Here's how the part is built. I have some questions about the finished solid (model axes, mm). Face numbers are marked on the shaded views. A direction names the side the tool comes from. Coordinates: 2 decimals unless noted, no trailing zeros. Loops run counter-clockwise (first coordinate to the right, second up) from the corner with the lowest first, then second, coordinate; pieces in that order, holes last. Notation, with made-up numbers: (0.5, -18) -> (41.5, -18) arc R9 cw to (41.5, -3) -> close; hole circle Ø7 at (42, 24). An arc over 180 degrees is marked (long way). Answer as a JSON object with one key per item and string values. Group by question number.
1) I need wall thicknesses on probe 1 along X at (y, z) = (-31, 39); probe 2 along Y at (x, z) = (14, 156.5); probe 3 along Y at (x, z) = (12, 41.5). Which ranges of each line are inside material? Lowest first, please. Write a range as [from, to].
2) I want a section at A-A (z = 48). Write out the boundary of the cut face in (x, y).
3) If we mould it in two halves opening along Y, with no side actions, what happens to the marked faces 1, 2 and 3? For each: +Y half, -Y half, draft (parallel to the pull), parting line (faces both ways), or undercut.
4) Which directions (+Z, -Z, +X, -X, +Y, -Y) give clear straight access to the entire face, cutting with the end or side of a thin tool? Please do the marked faces 4 and 5.
5) I want a section at B-B (x = 20). Write out the boundary of the cut face in (y, z), then the cut area to 3 significant figures.
6) I want a section at D-D (x = 38). Write out the boundary of the cut face in (y, z), then the cut area to 3 significant figures.
7) I want a section at C-C (y = 32). Write out the boundary of the cut face in (x, z), then the cut area to 4 significant figures.
8) I'm going to push a flat-ended pin straight in: pin 1 (10 mm diameter, centred on y = 1, z = 142, fed in from +X). Where does the tip first touch, or does it pass through?
Autodesk Inventor part; units mm, degrees
ref_plane "Начальная плоскость" through (0, 0, 23) normal (0, 0, 1) x (1, 0, 0)
ref_plane "Конечная плоскость" through (0, 0, 232) normal (0, 0, 1) x (1, 0, 0)
ref_plane "РабПлоскость8" through (-82, -50, 23) normal (0, 0, -1) x (-1, 0, 0)
ref_plane "Начальная плоскость" through (0, 0, 23) normal (0, 0, 1) x (1, 0, 0)
ref_plane "Конечная плоскость" through (0, 0, 232) normal (0, 0, 1) x (1, 0, 0)
sketch "Эскиз" plane through (0, 0, 0) normal (0, 0, 1) x (1, 0, 0)
  line L0 (46, -50) -> (0, -50)
  line L1 (46, -50) -> (46, -46.6496)
  line L2 (43.2392, -43.6591) -> (10.9418, -41.0753)
  line L3 (4.5, -34.0976) -> (4.5, 34.0976)
  line L4 (43.2392, 43.6591) -> (10.9418, 41.0753)
  line L5 (46, 46.6496) -> (46, 50)
  line L6 (0, 50) -> (46, 50)
  line L7 (0, -50) -> (0, 50)
  arc A0 (4.5, -34.0976) -> (10.9418, -41.0753) centre (11.5, -34.0976) ccw
  arc A1 (10.9418, 41.0753) -> (4.5, 34.0976) centre (11.5, 34.0976) ccw
  arc A2 (46, -46.6496) -> (43.2392, -43.6591) centre (43, -46.6496) ccw
  arc A3 (43.2392, 43.6591) -> (46, 46.6496) centre (43, 46.6496) ccw
  line L8 (0, 70) -> (0, -70) construction
  line L9 (-9.3169, 0) -> (55.9016, 0) construction
  point P0 (46, -43.88)
  point P1 (4.5, -40.56)
  point P2 (4.5, 40.56)
  point P3 (46, 43.88)
  dimension "d3" = 46
  dimension "d5" = 4.5
  dimension "d7" = 100
  dimension "d9" = 9.44
  dimension "d11" = 9.44
  dimension "d13" = 6.12
  dimension "d15" = 6.12
  dimension "d22" = 7
  dimension "d23" = 3
  dimension "d24" = 50
  dimension "d25" = 0
extrude "Тело" add sketch "Эскиз" along normal up to surface (209 mm away) from surface at 23
sketch "Sketch3" plane through (0, 0, 0) normal (0, 0, 1) x (1, 0, 0)
  line L0 (0, 0) -> (10, 0)
ref_plane "Work Plane7" through (0, 0, 0) normal (0, -1, 0) x (1, 0, 0)
sketch "Sketch4" plane through (0, 0, 0) normal (0, -1, 0) x (1, 0, 0)
  line L0 (-2, 23) -> (12, 23)
  line L1 (-2, 232) -> (12, 232)
  dimension "d29" = 209
ref_plane "РабПлоскость8" through (-82, -50, 23) normal (0, 0, -1) x (-1, 0, 0)
split "Разделение1" plane through (-82, -50, 23) removes the side toward (0, 0, -1)
ref_plane "РабПлоскость9" through (533, -50, 232) normal (0, 0, 1) x (1, 0, 0)
split "Разделение2" plane through (533, -50, 232) removes the side toward (0, 0, 1)
equation "\"d3\" = b"
equation "\"d7\" = ParH"
equation "\"d22\" = R"
equation "\"d23\" = R1"
equation "\"d24\" = 0.5 * d7"
equation "\"d16\" = G_L"
equation "\"R1\" = 3"
equation "\"R\" = 7"
equation "\"t1\" = 4.5"
equation "\"t2\" = 7.6"
equation "\"ParH\" = 100"
equation "\"b\" = 46"
equation "\"msp_x1\" = 0.04 * b"
equation "\"msp_x2\" = -0.08 * t1 + 0.04 * b"
equation "\"G_L\" = d29"
equation "\"ex\" = 0"
equation "\"G_OFFSET_START\" = -23"
equation "\"G_OFFSET_END\" = -23"
equation "\"d26\" = -G_OFFSET_START"
equation "\"d27\" = G_OFFSET_END + B_L"
equation "\"B_L\" = 255"
properties part number "Швеллер 10U-209 ГОСТ 8240-97" material "Сталь, мягкая, сварочная"
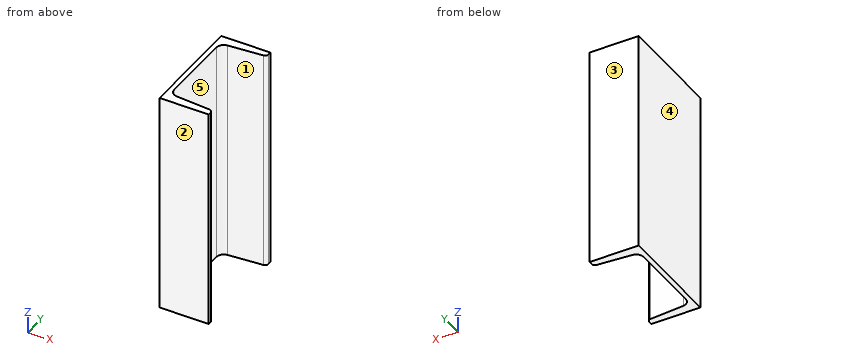
Determined:
{
 "1": {"probe 1": "[0, 4.5]", "probe 2": "[-50, -41.32], [41.32, 50]", "probe 3": "[-50, -41.16], [41.16, 50]"},
 "2": {"outline": "(0, -50) -> (46, -50) -> (46, -46.65) arc R3 ccw to (43.24, -43.66) -> (10.94, -41.08) arc R7 cw to (4.5, -34.1) -> (4.5, 34.1) arc R7 cw to (10.94, 41.08) -> (43.24, 43.66) arc R3 ccw to (46, 46.65) -> (46, 50) -> (0, 50) -> close"},
 "3": {"face 1": "undercut", "face 2": "-Y half", "face 3": "+Y half"},
 "4": {"face 4": "+Z, -Z, -X, +Y, -Y", "face 5": "+Z, -Z, +X"},
 "5": {"outline": "(-50, 23) -> (-41.8, 23) -> (-41.8, 232) -> (-50, 232) -> close; (41.8, 23) -> (50, 23) -> (50, 232) -> (41.8, 232) -> close", "area": "3,430 mm^2"},
 "6": {"outline": "(-50, 23) -> (-43.24, 23) -> (-43.24, 232) -> (-50, 232) -> close; (43.24, 23) -> (50, 23) -> (50, 232) -> (43.24, 232) -> close", "area": "2,830 mm^2"},
 "7": {"outline": "(0, 23) -> (4.5, 23) -> (4.5, 232) -> (0, 232) -> close", "area": "940.5 mm^2"},
 "8": {"pin 1": "x = 4.5"}
}
